Design review of the part built by this model. Coordinates are the model's own, in mm. A direction names the side the tool comes from. Round coordinates to 2 decimals unless told otherwise and drop trailing zeros. Loops run counter-clockwise (first coordinate to the right, second up) from the corner with the lowest first, then second, coordinate; pieces in that order, holes last. Notation, with made-up numbers: M 19,50.25 L 52,50.25 A19 ccw 52,72.25 Z; hole C -21,68.25 d7. An arc over 180 degrees is marked long. One line per item, written item: value. Start each with the question number.
Item 1: We need section C-C (y = 16). Write out the cut boundary in (x, z), then the cut area to 3 significant figures.
Item 2: We need section B-B (z = -37). Write out the cut boundary in (x, y).
Item 3: We need section A-A (y = 25). Write out the cut boundary in (x, z).
Item 4: For line 1 along X through (y, z) = (0.5, 0); line 2 along Z through (x, y) = (11, -11.5); line 3 along Z through (x, y) = (0, -12.5), list the stretches that pass through material, from the lowest coordinate up.
Item 5: We need section D-D (y = -36). Write out the cut boundary in (x, z).
Item 6: For faces 5 (the flat face through (-30, 25, -42)), 6 (the cylindrical face through (-21, 10, -28)), 7 (the cylindrical face through (1.32, 14.79, -29.97)), 8 (the flat face through (27, 20, 27)), 9 (the flat face through (-27, 20, 27)), list the 3-axis set-ups (+Z, -Z, +X, -X, +Y, -Y) from which the entire face can be reached by the end or side of a thin tool; tool diameter is ignored.
Item 7: Clearance check with flat-ended pins moving along their axes: pin 1 (5 mm diameter, centred on y = 26, z = -45.5, fed in from +X); pin 2 (17.5 mm diameter, centred on x = -14.5, z = 22, fed in from -Y); pin 3 (5 mm diameter, centred on x = 30, z = -29.6, fed in from -Y). State where each tip first meets the part, or that it passes through.
Item 8: Mouldability with a two-part tool opening along X and no side actions: class faces 1 (the flat face through (30, 25, -42)), 2 (the cylindrical face through (-33, 25, 34)), 3 (the cylindrical face through (-19.55, 25.07, -40.04)), 4 (the flat face through (0, 25, 35)) as released by +X, released by -X, zero draft, split by the parting line, or undercut.
from build123d import *

# Parameters (mm, degrees)
SKETCH1_R                = 35
SKETCH1_R_2              = 30
BOSS_EXTRUDE1_DEPTH      = 30
BOSS_EXTRUDE2_REACH      = 94.871
BOSS_EXTRUDE2_END_RADIUS = 35
SKETCH4_W                = 70
SKETCH4_H                = 10
SKETCH5_R                = 1.6
CUT_EXTRUDE1_DEPTH       = 95.074438611
FILLET1_R                = 5
SKETCH7_W                = 60
SKETCH7_H                = 10
BOSS_EXTRUDE3_DEPTH      = 15
SKETCH6_R                = 1.5
CUT_EXTRUDE2_DEPTH       = 15


# Read off the part's stored shape, not the designer's step: Split2
with BuildPart() as part:
    # Sketch1 → Boss-Extrude1 (new body)
    with BuildSketch(Plane(origin=(0, 0, 0), x_dir=(1, 0, 0), z_dir=(0, 1, 0))):
        with Locations(Location((0, 0, 0), (0, 0, 270))):
            Circle(SKETCH1_R)
        with Locations(Location((0, 0, 0), (0, 0, 270))):
            Circle(SKETCH1_R_2, mode=Mode.SUBTRACT)
    extrude(amount=BOSS_EXTRUDE1_DEPTH)

    # Sketch3 → Revolve1 (revolve)
    with BuildSketch(Plane.XY, mode=Mode.PRIVATE) as revolve1_sk:
        Polygon((2, -50), (35, 0), (30, 0), (2, -45), (0, -45), (0, -50), align=None)
    revolve(revolve1_sk.sketch.rotate(Axis((0, 0, 0), (0, -1, 0)), 180), axis=Axis((0, 0, 0), (0, -1, 0)))


with BuildPart() as body_2:
    # Split1: the piece on the far side of the plane
    add(part.part)
    split(bisect_by=Plane(origin=(0, 0, 0), x_dir=(0, 0, 1), z_dir=(1, 0, 0)), keep=Keep.BOTTOM)


with BuildPart() as part_1:
    add(part.part)

    # Split1
    split(bisect_by=Plane(origin=(0, 0, 0), x_dir=(0, 0, 1), z_dir=(1, 0, 0)), keep=Keep.TOP)

    add(body_2.part)  # Boss-Extrude2 merges body 2
    # Boss-Extrude2: up to this cylinder (the profile starts outside it)
    boss_extrude2_end = Plane(origin=(0, 25, 0), z_dir=(0, -1, 0)) * Cylinder(BOSS_EXTRUDE2_END_RADIUS, 260.742, mode=Mode.PRIVATE)
    # Sketch4 → Boss-Extrude2 (add, up to the surface)
    with BuildSketch(Plane(origin=(35, 0, 0), x_dir=(0, 0, -1), z_dir=(1, 0, 0)), mode=Mode.PRIVATE) as boss_extrude2_sk1:
        with Locations((0, 25)):
            Rectangle(SKETCH4_W, SKETCH4_H)
    boss_extrude2_tool1 = extrude(boss_extrude2_sk1.sketch, amount=-BOSS_EXTRUDE2_REACH, mode=Mode.PRIVATE) - boss_extrude2_end
    boss_extrude2 = boss_extrude2_tool1.solids().sort_by_distance((35, 25, 0))[0] + boss_extrude2_tool1.solids().sort_by_distance((35, 25, 0))[1]
    add(boss_extrude2)

    # Mirror1: Boss-Extrude2 across plane
    add(boss_extrude2.mirror(Plane(origin=(0, 0, 0), x_dir=(0, 0, 1), z_dir=(1, 0, 0))))

    # Sketch5 → Cut-Extrude1 (cut, through all)
    with BuildSketch(Plane(origin=(0, 30, 0), x_dir=(1, 0, 0), z_dir=(0, 1, 0))):
        with Locations(Location((-30, 29.59590276, 0), (0, 0, 270))):
            Circle(SKETCH5_R)
        with Locations(Location((30, 29.59590276, 0), (0, 0, 270))):
            Circle(SKETCH5_R)
    extrude(amount=-CUT_EXTRUDE1_DEPTH, mode=Mode.SUBTRACT)

    # Fillet1
    fillet1_edges = [part_1.edges().sort_by_distance(p)[0] for p in [
        (35, 25, -35),
        (35, 25, 35),
        (-35, 25, 35),
        (-35, 25, -35),
    ]]
    fillet(fillet1_edges, radius=FILLET1_R)


with BuildPart() as body_2_2:
    # Split2: the piece on the far side of the plane
    add(part_1.part)
    split(bisect_by=Plane.YZ, keep=Keep.BOTTOM)


with BuildPart() as part_2:
    add(part_1.part)

    # Split2
    split(bisect_by=Plane.YZ, keep=Keep.TOP)

    add(body_2_2.part)  # Boss-Extrude3 merges body 2 2
    # Sketch7 → Boss-Extrude3 (add)
    with BuildSketch(Plane(origin=(0, 0, -35), x_dir=(-1, 0, 0), z_dir=(0, 0, -1))):
        with Locations((0, 25)):
            Rectangle(SKETCH7_W, SKETCH7_H)
    extrude(amount=BOSS_EXTRUDE3_DEPTH)

    # Sketch6 → Cut-Extrude2 (cut)
    with BuildSketch(Plane(origin=(0, 30, 0), x_dir=(1, 0, 0), z_dir=(0, 1, 0))):
        with Locations(Location((-20, 41.471784691, 0), (0, 0, 270))):
            Circle(SKETCH6_R)
        with Locations(Location((20, 41.471784691, 0), (0, 0, 270))):
            Circle(SKETCH6_R)
    extrude(amount=-CUT_EXTRUDE2_DEPTH, mode=Mode.SUBTRACT)


solid = part_2.part
A:
1. outline: C 0,0 d70; hole C 0,0 d60
1. area: 1,020 mm2
2. outline: M -30,20 L 30,20 L 30,30 L -30,30 Z
3. outline: M -35,-30 A5 ccw -30,-35 L -30,-50 L 30,-50 L 30,-35 A5 ccw 35,-30 L 35,30 A5 ccw 30,35 L -30,35 A5 ccw -35,30 Z; hole C -30,-29.6 d3.2; hole C 0,0 d60; hole C -20,-41.47 d3; hole C 20,-41.47 d3; hole C 30,-29.6 d3.2
4. line 1: -35 to -30, 30 to 35
4. line 2: -25.11 to -20.02, 20.02 to 25.11
4. line 3: -26.75 to -22.22, 22.22 to 26.75
5. outline: C 0,0 d22.48; hole C 0,0 d15.2
6. face 5: -Z, -X, +Y, -Y
6. face 6: -Y
6. face 7: +Y
6. face 8: +Z, +X, -Y
6. face 9: +Z, -X, -Y
7. pin 1: x = 30
7. pin 2: y = -26.37
7. pin 3: y = 20
8. face 1: released by +X
8. face 2: released by -X
8. face 3: undercut
8. face 4: zero draft
